Source: CAD feature listing. Evaluate the final solid. Frame: model axes, mm. A direction names the side the tool comes from. Coordinates: 2 decimals unless noted, no trailing zeros. Loops run counter-clockwise (first coordinate to the right, second up) from the corner with the lowest first, then second, coordinate; pieces in that order, holes last. Notation, with made-up numbers: M -36,-6.5 L -2,-6.5 A7 ccw -2,6.5 Z; hole C -36.5,2 d11. An arc over 180 degrees is marked long. One line per question, with ' | ' between items. Start each with the question number.
1. Ray query, probe 1 along Z at (x, y) = (5, -9.05); probe 2 along Z at (x, y) = (-2, 5.5); probe 3 along Y at (x, z) = (8.75, 9). Return the intervals inside material, ascending.
2. Section query D-D, the plane y = 1. Output: boundary loops of the cut face in (x, z), and give its area (3 significant figures).
3. Section query B-B, the plane x = 4.25. Output: boundary loops of the cut face in (y, z), and give its area (3 significant figures).
4. Section query A-A, the plane z = 12. Output: boundary loops of the cut face in (x, y), and give its area (3 significant figures).
5. Mould query, pull axis Z, two halves, no side actions, for faces 1 (the cylindrical face through (-3.526, -9.486, 13.352)), 2 (the flat face through (0, 1, 2)), 3 (the cylindrical face through (-6.1, -1.2, 1)), 4 (the cylindrical face through (3.526, -9.486, 10.648)). Classes: pulls with the +Z half, pulls with the -Z half, needs draft (parallel to the pull), parting line crosses it, or undercut.
6. Access query for faces 5 (the flat face through (0, -8.5, 11)), 6 (the flat face through (0, 0, 0)). Directions: +Z, -Z, +X, -X, +Y, -Y. A direction counts if a zero-diameter tool reaches every point of the face in a straight line with its end or side. Return the directions, or none.
7. Pin query (flat end, axial travel): P1, Ø1.5, axis at x = -2.5, z = 5, coming from the +Y side; P2, Ø1.5, axis at x = 0.5, y = 2, coming from the +Z side. Return the tip coordinate at first contact, or that it passes through.
8. Section query C-C, the plane x = 0.5. Output: boundary loops of the cut face in (y, z).
```python
from build123d import *

# Parameters (mm, degrees)
SKETCH1_W           = 19
SKETCH1_H           = 21
BOSS_EXTRUDE1_DEPTH = 2
SKETCH3_W           = 19
SKETCH3_H           = 2
BOSS_EXTRUDE3_DEPTH = 19
SKETCH6_R           = 2
CUT_EXTRUDE1_DEPTH  = 2
SKETCH7_R           = 2
CUT_EXTRUDE2_DEPTH  = 2


with BuildPart() as part:
    # Sketch1 → Boss-Extrude1 (new body)
    with BuildSketch(Plane.XY):
        Rectangle(SKETCH1_W, SKETCH1_H)
    extrude(amount=BOSS_EXTRUDE1_DEPTH)

    # Sketch3 → Boss-Extrude3 (add)
    with BuildSketch(Plane.XY.offset(2)):
        with Locations((0, -9.5)):
            Rectangle(SKETCH3_W, SKETCH3_H)
    extrude(amount=BOSS_EXTRUDE3_DEPTH)

    # Sketch6 → Cut-Extrude1 (cut)
    with BuildSketch(Plane.XY.offset(2)):
        with Locations((-4.5, 0)):
            Circle(SKETCH6_R)
        with Locations(Location((4.5, 0, 0), (0, 0, 180))):
            Circle(SKETCH6_R)
    extrude(amount=-CUT_EXTRUDE1_DEPTH, mode=Mode.SUBTRACT)

    # Sketch7 → Cut-Extrude2 (cut)
    with BuildSketch(Plane(origin=(0, -8.5, 0), x_dir=(1, 0, 0), z_dir=(0, 1, 0))):
        with Locations(Location((-5, -12, 0), (0, 0, 180))):
            Circle(SKETCH7_R)
        with Locations((5, -12)):
            Circle(SKETCH7_R)
    extrude(amount=-CUT_EXTRUDE2_DEPTH, mode=Mode.SUBTRACT)


solid = part.part
```
Taken from the geometry:
1) probe 1: 0 to 10, 14 to 21 | probe 2: 0 to 2 | probe 3: -10.5 to -8.5
2) outline: M -9.5,0 L -6.23,0 L -6.23,2 L -9.5,2 Z; M -2.77,0 L 2.77,0 L 2.77,2 L -2.77,2 Z; M 6.23,0 L 9.5,0 L 9.5,2 L 6.23,2 Z | area: 24.1 mm^2
3) outline: M -10.5,0 L -1.98,0 L -1.98,2 L -8.5,2 L -8.5,10.15 L -10.5,10.15 Z; M -10.5,13.85 L -8.5,13.85 L -8.5,21 L -10.5,21 Z; M 1.98,0 L 10.5,0 L 10.5,2 L 1.98,2 Z | area: 64.6 mm^2
4) outline: M -9.5,-10.5 L -7,-10.5 L -7,-8.5 L -9.5,-8.5 Z; M -3,-10.5 L 3,-10.5 L 3,-8.5 L -3,-8.5 Z; M 7,-10.5 L 9.5,-10.5 L 9.5,-8.5 L 7,-8.5 Z | area: 22.0 mm^2
5) face 1: undercut | face 2: pulls with the +Z half | face 3: needs draft | face 4: undercut
6) face 5: +Z, +X, -X, +Y | face 6: -Z, +X, -X, +Y, -Y
7) P1: y = -8.5 | P2: z = 2
8) outline: M -10.5,0 L 10.5,0 L 10.5,2 L -8.5,2 L -8.5,21 L -10.5,21 Z
